```python
from build123d import *

# Parameters (mm, degrees)
SKETCH_1_W      = 18.2
SKETCH_1_H      = 13.2
SKETCH_1_W_2    = 9.4
SKETCH_1_H_2    = 4.7
EXTRUDE_1_DEPTH = 5
SKETCH_6_W      = 18.2
SKETCH_6_H      = 13.2
EXTRUDE_4_DEPTH = 1
SKETCH_7_W      = 1.4
SKETCH_7_H      = 10.2
EXTRUDE_5_DEPTH = 1


with BuildPart() as part:
    # Эскиз1 → Бобышка-Вытянуть1 (new body)
    with BuildSketch(Plane(origin=(0, 0, 0), x_dir=(1, 0, 0), z_dir=(0, 1, 0))):
        Rectangle(SKETCH_1_W, SKETCH_1_H)
        Polygon((-6.2, -5.1), (-6.2, 1.1), (6.2, 1.1), (6.2, -5.1), (7.6, -5.1), (7.6, 5.1), (-7.6, 5.1), (-7.6, -5.1), align=None, mode=Mode.SUBTRACT)
        with Locations((0, -2.75)):
            Rectangle(SKETCH_1_W_2, SKETCH_1_H_2, mode=Mode.SUBTRACT)
    extrude(amount=EXTRUDE_1_DEPTH)

    # Эскиз6 → Бобышка-Вытянуть4 (add)
    with BuildSketch(Plane.XZ):
        Rectangle(SKETCH_6_W, SKETCH_6_H)
    extrude(amount=EXTRUDE_4_DEPTH)

    # Эскиз7 → Бобышка-Вытянуть5 (add)
    with BuildSketch(Plane(origin=(0, 0, 0), x_dir=(1, 0, 0), z_dir=(0, 1, 0))):
        with Locations((-6.9, 0)):
            Rectangle(SKETCH_7_W, SKETCH_7_H)
        with Locations((6.9, 0)):
            Rectangle(SKETCH_7_W, SKETCH_7_H)
    extrude(amount=EXTRUDE_5_DEPTH)


solid = part.part
```
Design review of the part built by this model. Coordinates are the model's own, in mm. A direction names the side the tool comes from. Coordinates: 2 decimals unless noted, no trailing zeros. Order: outer loops, then holes, each group sorted by start corner. A loop starts at its lowest first (then second) coordinate and runs counter-clockwise, first axis right, second up. Notation, with made-up numbers: M 50.25,7 L 102.25,7 A18 ccw 102.25,33 Z; hole C 20.5,-39.5 d5. An arc over 180 degrees is marked long. Answer as a JSON object with one key per item and string values. Group by question number.
1) Add section A-A, the plane y = 0.65. Write out the cut boundary in (x, z).
2) Mouldability with a two-part tool opening along X and no side actions: class faces 1 (the flat face through (0, 0, -3)), 2 (the flat face through (0, -1, 0)), 3 (the flat face through (-9.1, 2, 0)) as pulls with the +X half, pulls with the -X half, needs draft (parallel to the pull), parting line crosses it, or undercut.
3) Add section C-C, the plane z = -3.5. Write out the cut boundary in (x, y), then the cut area to 3 significant figures.
4) For pin 1 (2.5 mm diameter, centred on x = 2, z = 2.5, fed in from +Y), flat-tipped, find the tip position at first contact; note if it passes through.
5) Tool access review of faces 4 (the flat face through (0, 2, 0.4)), 5 (the flat face through (0, 2, -6.6)): name each direction out of +Z, -Z, +X, -X, +Y, -Y from which nothing blocks a thin tool from reaching the whole face with its end or side.
6) Add section B-B, the plane x = 1. Write out the cut boundary in (y, z), then the cut area to 3 significant figures.
7) Wall thickness on L1, parallel to Z at x = -1.5, y = 3.55; L2, parallel to X at y = 4.5, z = 4.75; L3, parallel to X at y = 1.9, z = -2.25: over which ranges is each line inside the solid? List them lowest first.
8) Add section D-D, the plane z = 4. Write out the cut boundary in (x, y), then the cut area to 3 significant figures.
Computed values:
{
 "1": {"outline": "M -9.1,-6.6 L 9.1,-6.6 L 9.1,6.6 L -9.1,6.6 Z; hole M -6.2,-5.1 L 6.2,-5.1 L 6.2,-1.1 L -6.2,-1.1 Z; hole M -4.7,0.4 L 4.7,0.4 L 4.7,5.1 L -4.7,5.1 Z"},
 "2": {"face 1": "undercut", "face 2": "needs draft", "face 3": "pulls with the -X half"},
 "3": {"outline": "M -9.1,-1 L 9.1,-1 L 9.1,5 L 7.6,5 L 7.6,1 L 6.2,1 L 6.2,0 L -6.2,0 L -6.2,1 L -7.6,1 L -7.6,5 L -9.1,5 Z", "area": "36.0 mm^2"},
 "4": {"pin 1": "stops at y = 0"},
 "5": {"face 4": "+Y", "face 5": "-Z, +X, -X, +Y, -Y"},
 "6": {"outline": "M -1,-6.6 L 5,-6.6 L 5,-5.1 L 0,-5.1 L 0,-1.1 L 5,-1.1 L 5,0.4 L 0,0.4 L 0,5.1 L 5,5.1 L 5,6.6 L -1,6.6 Z", "area": "35.7 mm^2"},
 "7": {"L1": "z = -6.6 to -5.1, -1.1 to 0.4, 5.1 to 6.6", "L2": "x = -9.1 to -7.6, -6.2 to -4.7, 4.7 to 6.2, 7.6 to 9.1", "L3": "x = -9.1 to -7.6, 7.6 to 9.1"},
 "8": {"outline": "M -9.1,-1 L 9.1,-1 L 9.1,5 L 7.6,5 L 7.6,1 L 6.2,1 L 6.2,5 L 4.7,5 L 4.7,0 L -4.7,0 L -4.7,5 L -6.2,5 L -6.2,1 L -7.6,1 L -7.6,5 L -9.1,5 Z", "area": "51.0 mm^2"}
}
